Part model, mm, in its own coordinate system. A direction names the side the tool comes from. Give positions to 0.01 mm unless a question says otherwise; leave off trailing zeros. Order: outer loops, then holes, each group sorted by start corner. A loop starts at its lowest first (then second) coordinate and runs counter-clockwise, first axis right, second up. Notation, with made-up numbers: (-15.75, -9.5) -> (17.25, -9.5) arc R12 cw to (17.25, 12.5) -> close; hole circle Ø2 at (43, 22). An arc over 180 degrees is marked (long way). Write item = value, one per line. Start each with the question number.
(1) Two-plate mould, pull along X, no slides. Class faces 6 (the flat face through (168, 22, 2)), 7 (the flat face through (166, 5, 16)), 8 (the flat face through (170.5, 22, 1)): pulls with the +X half, pulls with the -X half, needs draft (parallel to the pull), parting line crosses it, or undercut.
(2) Probe line 1 along Z through (x, y) = (169.5, 25); line 2 along X through (y, z) = (22, 1); line 3 along Y through (x, z) = (166, 18.25). List the from-to ranges inside material, lowest first. Write a range as from..to.
(3) Saw through at A-A, the plane x = 170. List the corners of the cut face in (y, z), then the cut area to 3 significant figures.
(4) Saw through at B-B, the plane y = 22. List the corners of the cut face in (x, z), then the cut area to 3 significant figures.
(5) Flat gauge pins, fed straight in: pin 1 (1 mm diameter, centred on y = 23, z = 6, fed in from +X); pin 2 (1.5 mm diameter, centred on x = 166, y = 5, fed in from +Z); pin 3 (2.5 mm diameter, centred on x = 166.25, y = 4.5, fed in from -Z). Where does each tip first touch, or does it go through?
(6) Which spindle directions (+Z, -Z, +X, -X, +Y, -Y) get a long thin tool onto all of the face, cutting with end or side? Do faces 1 (the cylindrical face through (167.63, 38.925, 0.986)), 2 (the flat face through (170.5, 22, 14)), 3 (the flat face through (166, 22, 16)), 4 (the flat face through (163.5, 22, 5)), 5 (the flat face through (164, 22, 20)). Say none if no direction does.
(7) Saw through at C-C, the plane y = 17.5. List the corners of the cut face in (x, z), then the cut area to 3 significant figures.
(8) Saw through at D-D, the plane x = 165.5. State how many separate pieces and enclosed holes the cut face has, then the cut area to 3 significant figures.
from build123d import *

# Parameters (mm, degrees)
SKETCH040_W      = 11
SKETCH040_H      = 6
EXTRUDE014_DEPTH = 7
FILLET007_R      = 1
SKETCH031_W      = 8.5
SKETCH031_H      = 44
PAD003_DEPTH     = 20
SKETCH030_R      = 1.5
HOLE005_DEPTH    = 4
SKETCH033_R      = 1.5
HOLE007_DEPTH    = 4
SKETCH039_W      = 44
SKETCH039_H      = 6
POCKET001_DEPTH  = 7


with BuildPart() as part:
    # Sketch040 (on Face5 of Pocket001) → Extrude014 (new body)
    with BuildSketch(Plane.YZ.offset(163.5)):
        with Locations((30.5, 5)):
            Rectangle(SKETCH040_W, SKETCH040_H)
        with Locations((13.5, 5)):
            Rectangle(SKETCH040_W, SKETCH040_H)
    extrude(amount=EXTRUDE014_DEPTH)

    # Fillet007
    fillet007_edges = [part.edges().sort_by_distance(p)[0] for p in [
        (170.5, 8, 5),
        (170.5, 19, 5),
        (170.5, 36, 5),
        (170.5, 25, 5),
    ]]
    fillet(fillet007_edges, radius=FILLET007_R)

    # Sketch031 → Pad003 (new body)
    with BuildSketch(Plane.XY):
        with Locations((166.25, 22)):
            Rectangle(SKETCH031_W, SKETCH031_H)
    extrude(amount=PAD003_DEPTH)

    # Sketch030 → Hole005 (cut)
    with BuildSketch(Plane.XY):
        with Locations((166.244797, 39.500001)):
            Circle(SKETCH030_R)
        with Locations((166.247574, 22)):
            Circle(SKETCH030_R)
        with Locations((166.247574, 4.5)):
            Circle(SKETCH030_R)
    extrude(amount=HOLE005_DEPTH, mode=Mode.SUBTRACT)

    # Sketch033 (on Face5 of Hole005) → Hole007 (cut)
    with BuildSketch(Plane.XY.offset(20)):
        with Locations((166.244797, 39.500001)):
            Circle(SKETCH033_R)
        with Locations((166.247574, 22)):
            Circle(SKETCH033_R)
        with Locations((166.247574, 4.5)):
            Circle(SKETCH033_R)
    extrude(amount=-HOLE007_DEPTH, mode=Mode.SUBTRACT)

    # Sketch039 (on Face3 of Hole007) → Pocket001 (cut)
    with BuildSketch(Plane.YZ.offset(170.5)):
        with Locations((22, 5)):
            Rectangle(SKETCH039_W, SKETCH039_H)
    extrude(amount=-POCKET001_DEPTH, mode=Mode.SUBTRACT)


solid = part.part
Results list:
q1.face_6 = needs draft
q1.face_7 = undercut
q1.face_8 = pulls with the +X half
q2.line_1 = 0..2, 8..20
q2.line_2 = 162..164.75, 167.75..170.5
q2.line_3 = 0..3.02, 5.98..20.52, 23.48..38.02, 40.98..44
q3.outline = (0, 0) -> (44, 0) -> (44, 2) -> (0, 2) -> close; (0, 8) -> (44, 8) -> (44, 20) -> (0, 20) -> close
q3.area = 616 mm^2
q4.outline = (162, 0) -> (164.75, 0) -> (164.75, 2) -> (163.5, 2) -> (163.5, 8) -> (170.5, 8) -> (170.5, 20) -> (167.75, 20) -> (167.75, 16) -> (164.75, 16) -> (164.75, 20) -> (162, 20) -> close; (167.75, 0) -> (170.5, 0) -> (170.5, 2) -> (167.75, 2) -> close
q4.area = 110 mm^2
q5.pin_1 = 163.5
q5.pin_2 = 16
q5.pin_3 = 8
q6.face_1 = -Z
q6.face_2 = +Z, -Z, +X, +Y, -Y
q6.face_3 = +Z
q6.face_4 = +X, +Y, -Y
q6.face_5 = +Z, +X, -X, +Y, -Y
q7.outline = (162, 0) -> (170.5, 0) -> (170.5, 2) -> (163.5, 2) -> (163.5, 8) -> (170.5, 8) -> (170.5, 20) -> (162, 20) -> close
q7.area = 128 mm^2
q8.separate_pieces = 5
q8.enclosed_holes = 0
q8.area = 569 mm^2
